Input: dimensioned drawing with shaded views. Units: mm. Origin: part minimum x, y, z. A direction names the side the tool comes from. Give positions to 0.01 mm unless a question says otherwise; leave off trailing zeros. Write each loop counter-clockwise with the first axis right and the second up, starting at its lowest first coordinate (ties: lowest second). Pieces come first, ordered by that corner, then holes.
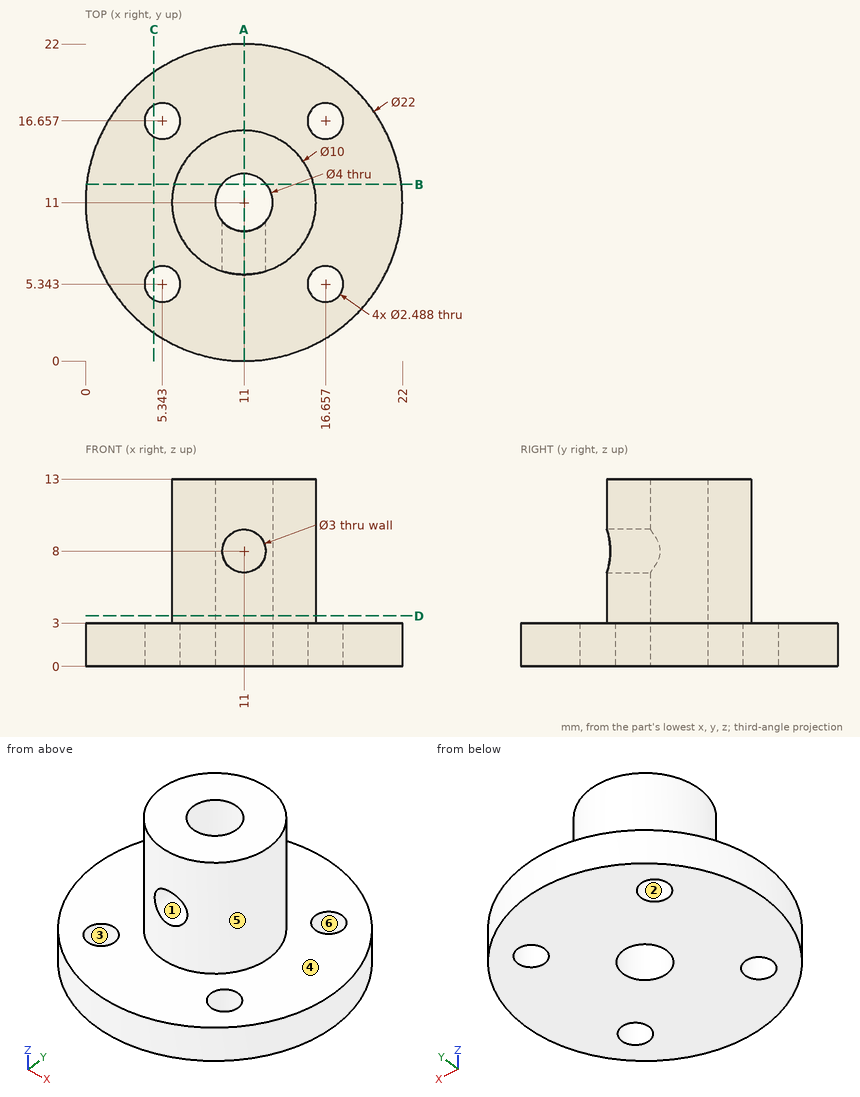
1. Cut plane C-C, the plane x = 4.75. Return the cut outline in (y, z), then the cut area to 3 significant figures.
2. Contact query for flat-ended pins moving along their axis: P1, Ø2, axis at x = 16.66, y = 5.34, coming from the +Z side; P2, Ø1.5, axis at x = 13, z = 3.5, coming from the -Y side (1 decimal); P3, Ø4, axis at x = 11, z = 8, coming from the -Y side; P4, Ø3, axis at x = 15.5, y = 2.5, coming from the +Z side. Output: stop coordinate, or through.
3. Line query: L1, parallel to Z at x = 11, y = 8.6; L2, parallel to X at y = 6, z = 1; L3, parallel to Y at x = 10.5, z = 2. Output: solid intervals per line, ascending.
4. Cut plane A-A, the plane x = 11. Return the cut outline in (y, z), then the cut area to 3 significant figures.
5. Mould query, pull axis X, two halves, no side actions, for the marked faces 3, 4, 5 and 6. Classes: +X half, -X half, draft (parallel to the pull), parting line (faces both ways), or undercut.
6. Access query for the marked faces 1 and 2. Directions: +Z, -Z, +X, -X, +Y, -Y. A direction counts if a zero-diameter tool reaches every point of the face in a straight line with its end or side. Return the directions, or none.
7. Cut plane B-B, the plane y = 12.25. Return the cut outline in (x, z).
8. Cut plane D-D, the plane z = 3.5. Return the cut outline in (x, y).
Response values:
1. outline: (1.95, 0) - (4.25, 0) - (4.25, 3) - (1.95, 3) - close; (6.44, 0) - (15.56, 0) - (15.56, 3) - (6.44, 3) - close; (17.75, 0) - (20.05, 0) - (20.05, 3) - (17.75, 3) - close
1. area: 41.2 mm2
2. P1: passes through
2. P2: stops at y = 0.1
2. P3: stops at y = 6
2. P4: stops at z = 3
3. L1: z = 0 to 6.5, 9.5 to 13
3. L2: x = 1.2 to 4.29, 6.4 to 15.6, 17.71 to 20.8
3. L3: y = 0.01 to 9.06, 12.94 to 21.99
4. outline: (0, 0) - (9, 0) - (9, 6.5) - (6, 6.5) - (6, 3) - (0, 3) - close; (6, 9.5) - (9, 9.5) - (9, 13) - (6, 13) - close; (13, 0) - (22, 0) - (22, 3) - (16, 3) - (16, 13) - (13, 13) - close
4. area: 105 mm2
5. face 3: undercut
5. face 4: draft
5. face 5: parting line
5. face 6: undercut
6. face 1: -Y
6. face 2: +Z, -Z
7. outline: (0.07, 0) - (9.44, 0) - (9.44, 13) - (6.16, 13) - (6.16, 3) - (0.07, 3) - close; (12.56, 0) - (21.93, 0) - (21.93, 3) - (15.84, 3) - (15.84, 13) - (12.56, 13) - close
8. outline: circle Ø10 at (11, 11); hole circle Ø4 at (11, 11)
